```python
from build123d import *

# Parameters (mm, degrees)
SKETCH1_R           = 2.5
BOSS_EXTRUDE1_DEPTH = 482.6
SKETCH2_W           = 61.361470627
SKETCH2_H           = 380.25471835
CUT_EXTRUDE1_DEPTH  = 21


with BuildPart() as part:
    # Sketch1 → Boss-Extrude1 (new body)
    with BuildSketch(Plane.XY):
        with BuildLine():
            Line((-5.63, 10), (-9, 10))
            ThreePointArc((-9, 10), (-9.707106781, 9.707106781), (-10, 9))
            Line((-10, 9), (-10, 5.63))
            Line((-10, 5.63), (-10, 3.6))
            Line((-10, 3.6), (-8.5, 3.6))
            Line((-8.5, 3.6), (-8.5, 5.63))
            Line((-8.5, 5.63), (-6.402046573, 5.63))
            Line((-6.402046573, 5.63), (-3.95, 3.177953427))
            Line((-3.95, 3.177953427), (-3.95, -3.088580227))
            Line((-3.95, -3.088580227), (-6.491419773, -5.63))
            Line((-6.491419773, -5.63), (-8.5, -5.63))
            Line((-8.5, -5.63), (-8.5, -3.6))
            Line((-8.5, -3.6), (-10, -3.6))
            Line((-10, -3.6), (-10, -5.63))
            Line((-10, -5.63), (-10, -9))
            ThreePointArc((-10, -9), (-9.707106781, -9.707106781), (-9, -10))
            Line((-9, -10), (-5.63, -10))
            Line((-5.63, -10), (-3.6, -10))
            Line((-3.6, -10), (-3.6, -8.5))
            Line((-3.6, -8.5), (-5.63, -8.5))
            Line((-5.63, -8.5), (-5.63, -6.402046573))
            Line((-5.63, -6.402046573), (-3.177953427, -3.95))
            Line((-3.177953427, -3.95), (2.991333041, -3.95))
            Line((2.991333041, -3.95), (5.63, -6.588666959))
            Line((5.63, -6.588666959), (5.63, -8.5))
            Line((5.63, -8.5), (3.6, -8.5))
            Line((3.6, -8.5), (3.6, -10))
            Line((3.6, -10), (5.63, -10))
            Line((5.63, -10), (9, -10))
            ThreePointArc((9, -10), (9.707106781, -9.707106781), (10, -9))
            Line((10, -9), (10, -5.63))
            Line((10, -5.63), (10, -3.6))
            Line((10, -3.6), (8.5, -3.6))
            Line((8.5, -3.6), (8.5, -5.63))
            Line((8.5, -5.63), (6.491419773, -5.63))
            Line((6.491419773, -5.63), (3.95, -3.088580227))
            Line((3.95, -3.088580227), (3.95, 3.177953427))
            Line((3.95, 3.177953427), (6.402046573, 5.63))
            Line((6.402046573, 5.63), (8.5, 5.63))
            Line((8.5, 5.63), (8.5, 3.6))
            Line((8.5, 3.6), (10, 3.6))
            Line((10, 3.6), (10, 5.63))
            Line((10, 5.63), (10, 9))
            ThreePointArc((10, 9), (9.707106781, 9.707106781), (9, 10))
            Line((9, 10), (5.63, 10))
            Line((5.63, 10), (3.6, 10))
            Line((3.6, 10), (3.6, 8.5))
            Line((3.6, 8.5), (5.63, 8.5))
            Line((5.63, 8.5), (5.63, 6.588666959))
            Line((5.63, 6.588666959), (2.991333041, 3.95))
            Line((2.991333041, 3.95), (-3.177953427, 3.95))
            Line((-3.177953427, 3.95), (-5.63, 6.402046573))
            Line((-5.63, 6.402046573), (-5.63, 8.5))
            Line((-5.63, 8.5), (-3.6, 8.5))
            Line((-3.6, 8.5), (-3.6, 10))
            Line((-3.6, 10), (-5.63, 10))
        make_face()
        Circle(SKETCH1_R, mode=Mode.SUBTRACT)
    extrude(amount=BOSS_EXTRUDE1_DEPTH)

    # Sketch2 → Cut-Extrude1 (cut, through all)
    with BuildSketch(Plane(origin=(0, 10, 0), x_dir=(1, 0, 0), z_dir=(0, 1, 0))):
        with Locations((14.074869471, -342.527359175)):
            Rectangle(SKETCH2_W, SKETCH2_H)
    extrude(amount=-CUT_EXTRUDE1_DEPTH, mode=Mode.SUBTRACT)


solid = part.part
```
Read the model definition and answer for the solid it produces. Units are mm, in the model's axes. A direction names the side the tool comes from. Round coordinates to 2 decimals unless told otherwise and drop trailing zeros. Write each loop counter-clockwise with the first axis right and the second up, starting at its lowest first coordinate (ties: lowest second). Pieces come first, ordered by that corner, then holes. Notation, with made-up numbers: M 62,64.5 L 96,64.5 A29 ccw 96,97.5 Z; hole C 13.25,77.25 d8. An arc over 180 degrees is marked long. One line per item, written item: value.
Q1. Find section A-A on x = 0. Write down the section's boundary in (y, z).
Data:
outline: M -3.95,0 L -2.5,0 L -2.5,152.4 L -3.95,152.4 Z; M 2.5,0 L 3.95,0 L 3.95,152.4 L 2.5,152.4 Z
Q2. Straight lines are drawn through the part: line 1 (X direction, y = 7.5, z = 39.5); line 2 (X direction, y = 0, z = 38). For each, find the intervals that lie inside material, in ascending order. Write a range as [from, to].
Data:
line 1: [-10, -5.63], [5.63, 10]
line 2: [-3.95, -2.5], [2.5, 3.95]
Q3. For a pull along X with two mould halves and no side action, classify faces 4 (the flat face through (-5.2, -4.34, 75.13)), 5 (the flat face through (-6, 10, 75)), 6 (the flat face through (-3.95, 0, 75)) as +X half, -X half, draft (parallel to the pull), parting line (faces both ways), or undercut.
Data:
face 4: undercut
face 5: draft
face 6: -X half
Q4. Flat-ended cylindrical pins translate along their axes: pin 1 Ø1.6 at (y, z) = (9.5, 103.5) entering from +X; pin 2 Ø1.9 at (x, z) = (1, 39.5) entering from -Y; pin 3 Ø0.8 at (x, z) = (-9.5, 93) entering from +Y (3 decimals); pin 4 Ø1.9 at (y, z) = (1, 89.5) entering from -X. Find the tip coordinate at first contact, or state that the pin passes through.
Data:
pin 1: x = 10
pin 2: y = -3.95
pin 3: y = 9.995
pin 4: x = -3.95
Q5. Which of the six approach directions +Z, -Z, +X, -X, +Y, -Y give full straight-line access (tool end or side, diameter ignored) to faces 1 (the flat face through (0, 3.95, 75)), 2 (the flat face through (4.33, 5.29, 75.13)), 3 (the flat face through (0, -3.95, 75))?
Data:
face 1: +Z, -Z, +Y
face 2: +Z, -Z
face 3: +Z, -Z, -Y
